from build123d import *

# Parameters (mm, degrees)
F0_W     = 120
F0_H     = 120
F0_R     = 3.5
F1_DEPTH = 7
F2_R     = 3
F3_R     = 3.5
F4_DEPTH = 25
F5_R     = 5.5
F6_DEPTH = 2


with BuildPart() as f1:
    # F0 (on Front) → F1 (new body)
    with BuildSketch(Plane.XZ):
        Rectangle(F0_W, F0_H)
        with Locations((-50, -50)):
            Circle(F0_R, mode=Mode.SUBTRACT)
        with Locations((50, -50)):
            Circle(F0_R, mode=Mode.SUBTRACT)
        with Locations((-50, 50)):
            Circle(F0_R, mode=Mode.SUBTRACT)
        with Locations((50, 50)):
            Circle(F0_R, mode=Mode.SUBTRACT)
    extrude(amount=F1_DEPTH)

    # F2
    f2_edges = [f1.edges().sort_by_distance(p)[0] for p in [
        (-60, -3.5, 60),
        (-60, -3.5, -60),
        (60, -3.5, -60),
        (60, -3.5, 60),
    ]]
    fillet(f2_edges, radius=F2_R)

    # F3 (on face) → F4 (cut)
    with BuildSketch(Plane(origin=(0, 0, 0), x_dir=(-1, 0, 0), z_dir=(0, 1, 0))):
        with Locations((-21.5, 40)):
            Circle(F3_R)
        with Locations((21.5, 40)):
            Circle(F3_R)
        with Locations((-21.5, -40)):
            Circle(F3_R)
        with Locations((21.5, -40)):
            Circle(F3_R)
    extrude(amount=-F4_DEPTH, mode=Mode.SUBTRACT)

    # F5 (on face) → F6 (cut)
    with BuildSketch(Plane(origin=(0, 0, 0), x_dir=(-1, 0, 0), z_dir=(0, 1, 0))):
        with Locations((-21.5, 40)):
            Circle(F5_R)
        with Locations((21.5, 40)):
            Circle(F5_R)
        with Locations((-21.5, -40)):
            Circle(F5_R)
        with Locations((21.5, -40)):
            Circle(F5_R)
    extrude(amount=-F6_DEPTH, mode=Mode.SUBTRACT)


solid = f1.part
Model file for the job. Use its own axes, mm. A direction names the side the tool comes from. Coordinates: 2 decimals unless noted, no trailing zeros. Order: outer loops, then holes, each group sorted by start corner. A loop starts at its lowest first (then second) coordinate and runs counter-clockwise, first axis right, second up. Notation, with made-up numbers: (-5, -12.75) -> (44, -12.75) arc R13 cw to (44, 10.25) -> close; hole circle Ø3 at (47.5, 14.25). An arc over 180 degrees is marked (long way). Return JSON: item names as keys, results as strings. Group by question number.
Item 1: Flat gauge pins, fed straight in: P1, Ø11, axis at x = -50, z = -50, coming from the +Y side; P2, Ø3.5, axis at x = 21.5, z = -38, coming from the +Y side. Where does each tip first touch, or does it go through?
Item 2: Saw through at C-C on x = -50. Write the cut outline in (y, z), then the cut area to 3 significant figures.
Item 3: Tool access for faces 1 (the cylindrical face through (47.42, -3.451, 52.365)), 2 (the flat face through (22, -2, 36)): list every direction of +Z, -Z, +X, -X, +Y, -Y with a clear straight run to the whole face (end or side of a thin tool).
Item 4: Saw through at B-B on y = -4.5. State how many separate pieces and enclosed holes the cut face has, then the cut area to 3 significant figures.
Item 5: Pull direction Z, two halves, no side cores. Call faces 3 (the flat face through (-60, -3, -1)), 4 (the cylindrical face through (-21.04, -4.46, 43.47)), 5 (the cylindrical face through (59.1, -3.55, -59.14)), 6 (the flat face through (-1, -3, 60)): pulls with the +Z half, pulls with the -Z half, needs draft (parallel to the pull), parting line crosses it, or undercut.
Item 6: Saw through at A-A on z = 40. Write the cut outline in (x, y).
Item 7: Wall check: line 1 along Z through (x, y) = (21.5, -4.7); line 2 along Z through (x, y) = (50, -5.25); line 3 along X through (y, z) = (-2.25, 38.5). Give the ranges that are in metal, low to high. Write a range as [from, to].
Item 8: Saw through at D-D on x = -21.5. Write the cut outline in (y, z), then the cut area to 3 significant figures.
Values found:
{
 "1": {"P1": "stops at y = 0", "P2": "stops at y = -2"},
 "2": {"outline": "(-7, -60) -> (0, -60) -> (0, -53.5) -> (-7, -53.5) -> close; (-7, -46.5) -> (0, -46.5) -> (0, 46.5) -> (-7, 46.5) -> close; (-7, 53.5) -> (0, 53.5) -> (0, 60) -> (-7, 60) -> close", "area": "742 mm2"},
 "3": {"face 1": "+Y, -Y", "face 2": "+Y"},
 "4": {"separate pieces": "1", "enclosed holes": "8", "area": "14,100 mm2"},
 "5": {"face 3": "needs draft", "face 4": "undercut", "face 5": "pulls with the -Z half", "face 6": "pulls with the +Z half"},
 "6": {"outline": "(-60, -7) -> (-25, -7) -> (-25, -2) -> (-27, -2) -> (-27, 0) -> (-60, 0) -> close; (-18, -7) -> (18, -7) -> (18, -2) -> (16, -2) -> (16, 0) -> (-16, 0) -> (-16, -2) -> (-18, -2) -> close; (25, -7) -> (60, -7) -> (60, 0) -> (27, 0) -> (27, -2) -> (25, -2) -> close"},
 "7": {"line 1": "z = [-60, -43.5], [-36.5, 36.5], [43.5, 60]", "line 2": "z = [-60, -53.5], [-46.5, 46.5], [53.5, 60]", "line 3": "x = [-60, -24.66], [-18.34, 18.34], [24.66, 60]"},
 "8": {"outline": "(-7, -60) -> (0, -60) -> (0, -45.5) -> (-2, -45.5) -> (-2, -43.5) -> (-7, -43.5) -> close; (-7, -36.5) -> (-2, -36.5) -> (-2, -34.5) -> (0, -34.5) -> (0, 34.5) -> (-2, 34.5) -> (-2, 36.5) -> (-7, 36.5) -> close; (-7, 43.5) -> (-2, 43.5) -> (-2, 45.5) -> (0, 45.5) -> (0, 60) -> (-7, 60) -> close", "area": "726 mm2"}
}
